The model under review builds one solid part; all positions refer to its coordinate system, in mm. A direction names the side the tool comes from. Coordinates: 2 decimals unless noted, no trailing zeros. Order: outer loops, then holes, each group sorted by start corner. A loop starts at its lowest first (then second) coordinate and runs counter-clockwise, first axis right, second up. Notation, with made-up numbers: M 5,59.5 L 50,59.5 A14 ccw 50,85.5 Z; hole C 62,40.5 d9. An arc over 180 degrees is marked long. Write each question's results on one line, items separated by ' | '.
Autodesk Inventor part; units mm, degrees
ref_plane "YZ Plane" through (0, 0, 0) normal (1, 0, 0) x (0, 1, 0)
ref_plane "XZ Plane" through (0, 0, 0) normal (0, 1, 0) x (-1, 0, 0)
ref_plane "XY Plane" through (0, 0, 0) normal (0, 0, 1) x (1, 0, 0)
sketch "Sketch1" plane through (0, 0, 0) normal (0, 1, 0) x (-1, 0, 0)
  line L0 (0, -4.826) -> (0, -37.338)
  line L1 (4.826, -42.164) -> (58.674, -42.164)
  line L2 (63.5, -37.338) -> (63.5, -4.826)
  line L3 (58.674, 0) -> (4.826, 0)
  arc A0 (4.826, 0) -> (0, -4.826) centre (4.826, -4.826) ccw
  arc A1 (63.5, -4.826) -> (58.674, 0) centre (58.674, -4.826) ccw
  arc A2 (58.674, -42.164) -> (63.5, -37.338) centre (58.674, -37.338) ccw
  arc A3 (0, -37.338) -> (4.826, -42.164) centre (4.826, -37.338) ccw
  circle A4 centre (4.826, -4.826) radius 4.826
  circle A5 centre (4.826, -37.338) radius 4.826
  circle A6 centre (58.674, -37.338) radius 4.826
  circle A7 centre (58.674, -4.826) radius 4.826
  circle A8 centre (58.674, -4.826) radius 2.3812
  circle A9 centre (58.674, -37.338) radius 2.3812
  circle A10 centre (4.826, -37.338) radius 2.3812
  circle A11 centre (4.826, -4.826) radius 2.3813
  point P0 (0, 0)
  point P1 (0, -42.164)
  point P2 (63.5, -42.164)
  dimension "d0" = 42.164
  dimension "d1" = 63.5
  dimension "d2" = 4.826
  dimension "d3" = 4.7625
  dimension "d4" = 4.7625
  dimension "d5" = 4.7625
extrude "Extrusion1" add sketch "Sketch1" against normal blind 4.7625
sketch "Sketch2" plane through (0, -4.7625, 0) normal (0, -1, 0) x (1, 0, 0)
  line L0 (0, -37.338) -> (0, -4.826)
  line L1 (0, -21.082) -> (-63.5, -21.082)
  line L2 (-63.5, -4.826) -> (-63.5, -37.338)
  line L3 (-58.674, -42.164) -> (-4.826, -42.164)
  line L4 (-31.75, -42.164) -> (-31.75, 0)
  circle A0 centre (-31.75, -21.082) radius 11.176
  line L5 (-31.75, -21.082) -> (-16.2142, -5.5462)
  line L6 (-31.75, -21.082) -> (-9.779, -21.082) construction
  line L7 (-31.75, -21.082) -> (-47.2858, -5.5462)
  line L8 (-47.2858, -5.5462) -> (-31.75, -21.082)
  line L9 (-31.75, -21.082) -> (-47.2858, -36.6178)
  line L10 (-47.2858, -36.6178) -> (-31.75, -21.082)
  line L11 (-31.75, -21.082) -> (-16.2142, -36.6178)
  circle A1 centre (-16.2142, -5.5462) radius 1.27
  circle A2 centre (-16.2142, -36.6178) radius 1.27
  circle A3 centre (-47.2858, -36.6178) radius 1.27
  circle A4 centre (-47.2858, -5.5462) radius 1.27
  point P0 (0, 0)
  dimension "d8" = 22.352
  dimension "d9" = 21.971
  dimension "d10" = 45
  dimension "d11" = 21.971
  dimension "d12" = 21.971
  dimension "d13" = 2.54
  dimension "d14" = 2.54
  dimension "d15" = 2.54
  dimension "d16" = 2.54
extrude "Extrusion2" cut sketch "Sketch2" against normal blind 21.971
sketch "Sketch3" plane through (0, -4.7625, 0) normal (0, -1, 0) x (1, 0, 0)
  point P0 (0, 0)
sketch "Sketch4" plane through (0, 0, 0) normal (0, 1, 0) x (1, 0, 0)
  line L0 (0, 4.826) -> (0, 37.338)
  line L1 (0, 21.082) -> (0, 15.367)
  line L2 (0, 15.367) -> (0, 21.082)
  line L3 (0, 21.082) -> (0, 26.797)
  line L4 (0, 15.367) -> (7.62, 15.367)
  line L5 (7.62, 15.367) -> (7.62, 26.797)
  line L6 (7.62, 26.797) -> (0, 26.797)
  line L7 (7.62, 15.367) -> (0, 7.747)
  line L8 (7.62, 15.367) -> (18.3963, 15.367) construction
  line L9 (7.62, 26.797) -> (0, 34.417)
  line L10 (0, 15.367) -> (-6.35, 15.367)
  line L11 (-6.35, 15.367) -> (-6.35, 26.797)
  line L12 (-6.35, 26.797) -> (0, 26.797)
  point P0 (0, 0)
  dimension "d19" = 5.715
  dimension "d20" = 5.715
  dimension "d21" = 7.62
  dimension "d22" = 135
  dimension "d23" = 6.35
extrude "Extrusion3" add sketch "Sketch4" against normal blind 4.7625 contours L0 L4 L7 | L6 L0 L9
extrude "Extrusion4" add sketch "Sketch4" against normal blind 9.525 contours L10 L11 L12 L0 | L0 L6 L5 L4
sketch "Sketch5" plane through (7.62, 0, -15.367) normal (1, 0, 0) x (0, 0, -1)
  line L0 (11.43, -4.7625) -> (0, -4.7625)
  line L1 (5.715, -4.7625) -> (5.715, -12.3825)
  circle A0 centre (5.715, -12.3825) radius 5.715
  point P0 (-15.367, 0)
  dimension "d28" = 7.62
  dimension "d29" = 11.43
extrude "Extrusion5" cut sketch "Sketch5" against normal blind 9.9441
sketch "Sketch6" plane through (0, 0, 0) normal (0, 1, 0) x (1, 0, 0)
  circle A0 centre (-16.2142, 5.5462) radius 1.27
  circle A1 centre (-16.2142, 5.5462) radius 1.5875
  circle A2 centre (-47.2858, 5.5462) radius 1.27
  circle A3 centre (-47.2858, 5.5462) radius 1.5875
  circle A4 centre (-47.2858, 36.6178) radius 1.27
  circle A5 centre (-47.2858, 36.6178) radius 1.5875
  circle A6 centre (-16.2142, 36.6178) radius 1.27
  circle A7 centre (-16.2142, 36.6178) radius 1.5875
  point P0 (0, 0)
  dimension "d46" = 3.175
  dimension "d47" = 3.175
  dimension "d48" = 3.175
  dimension "d49" = 3.175
extrude "Extrusion6" cut sketch "Sketch6" against normal up to surface (4.7625 mm away)
sketch "Sketch7" plane through (-6.35, -9.525, -26.797) normal (-1, 0, 0) x (0, 0, 1)
  line L0 (0, 4.7625) -> (0, 0)
  line L1 (0, 4.7625) -> (11.43, 4.7625)
  line L2 (0, 0) -> (11.43, 0)
  line L3 (11.43, 0) -> (11.43, 4.7625)
  line L4 (11.43, 4.7625) -> (0, 4.7625)
  line L5 (0, 4.7625) -> (0, 0)
  point P0 (26.797, 9.525)
extrude "Extrusion7" cut sketch "Sketch7" against normal up to surface (13.97 mm away)
equation "\"d17\" = d9"
properties part number "MotorTop_3DPrint"
1) Take a section at C-C on y = -0.85. Count the separate pieces of the cut face and the enclosed holes in it, plus the area to 3 significant figures.
Solutions:
separate pieces: 1 | enclosed holes: 9 | area: 2,310 mm2
2) Take a section at B-B on z = -20. State the section outline as (x, y) points.
Solutions:
outline: M -63.5,-4.76 L -42.87,-4.76 L -42.87,0 L -63.5,0 Z; M -20.63,-4.76 L 7.62,-4.76 L 7.62,0 L -20.63,0 Z
3) The part is to be moulded in two halves that separate along Z. For faces 1 (the cylindrical face through (-48.87, -2.35, -5.62)), 2 (the cylindrical face through (-62.12, -2.35, -1.45)), 3 (the flat face through (-20, 0, -21)), say which applies: pulls with the +Z half, pulls with the -Z half, needs draft (parallel to the pull), parting line crosses it, or undercut.
Solutions:
face 1: undercut | face 2: pulls with the +Z half | face 3: needs draft
4) Take a section at A-A on x = -31.75. State the section outline as (y, z) points, plus the area to 3 significant figures.
Solutions:
outline: M -4.76,-42.16 L 0,-42.16 L 0,-32.26 L -4.76,-32.26 Z; M -4.76,-9.91 L 0,-9.91 L 0,0 L -4.76,0 Z | area: 94.4 mm2
5) For pin 1 (1 mm diameter, centred on y = -2, z = -13, fed in from +X); pin 2 (18 mm diameter, centred on x = -31.75, z = -21.082, fed in from -Y); pin 3 (1.5 mm diameter, centred on y = -1.5, z = -6.5, fed in from +X), all flat-tipped, find the tip position at first contact; note any pin that passes through.
Solutions:
pin 1: x = 5.75 | pin 2: through | pin 3: x = 0
6) To check wall thickness, follow line 1 along Z through (x, y) = (-59, -2.45); line 2 along X through (y, z) = (-1.85, -5); line 3 along Z through (x, y) = (-57.5, -2.95). State the ranges of each line that lie inside material, in increasing order.
Solutions:
line 1: -42.15 to -39.7, -34.98 to -7.18, -2.47 to -0.01 | line 2: -63.5 to -61.05, -56.3 to -48.78, -45.8 to -17.7, -14.72 to -7.2, -2.45 to 0 | line 3: -42.16 to -39.41, -35.27 to -6.9, -2.75 to 0
7) For faces 4 (the cylindrical face through (-21.426, -2.415, -25.362)), 5 (the flat face through (0, -2, -6)), list the 3-axis set-ups (+Z, -Z, +X, -X, +Y, -Y) from which the entire face can be reached by the end or side of a thin tool; tool diameter is ignored.
Solutions:
face 4: +Y, -Y | face 5: +Z, +X, +Y, -Y
8) Take a section at D-D on z = -39. State the section outline as (x, y) points.
Solutions:
outline: M -63.2,-4.76 L -60.38,-4.76 L -60.38,0 L -63.2,0 Z; M -56.97,-4.76 L -6.53,-4.76 L -6.53,0 L -56.97,0 Z; M -3.12,-4.76 L -0.3,-4.76 L -0.3,0 L -3.12,0 Z
